```python
from build123d import *

# Parameters (mm, degrees)
F0_W     = 103.353604
F0_H     = 45.458422
F1_DEPTH = 25.4
F2_R     = 12.877415
F3_R     = 21.377303
F4_DEPTH = 27.686


with BuildPart() as f1:
    # F0 (on Top) → F1 (new body)
    with BuildSketch(Plane.XY):
        Rectangle(F0_W, F0_H)
    extrude(amount=F1_DEPTH)

    # F2
    f2_edges = [f1.edges().sort_by_distance(p)[0] for p in [
        (51.676802, 22.729211, 12.7),
        (51.676802, -22.729211, 12.7),
    ]]
    fillet(f2_edges, radius=F2_R)

    # F3 (on Top) → F4 (join)
    with BuildSketch(Plane.XY):
        with Locations((-21.615615, 0)):
            Circle(F3_R)
    extrude(amount=-F4_DEPTH)


solid = f1.part
```
The listing builds one solid part. Answer for the finished solid, in the listing's coordinates (mm). A direction names the side the tool comes from. Round coordinates to 2 decimals unless told otherwise and drop trailing zeros. Loops run counter-clockwise (first coordinate to the right, second up) from the corner with the lowest first, then second, coordinate; pieces in that order, holes last.
Q1. Section C-C, the plane x = -28.5 is taken. Determine the outline of the cut face in (y, z), then the cut area to 3 significant figures.
Q2. Section B-B, the plane z = -9 is taken. Determine the outline of the cut face in (x, y), then the cut area to 3 significant figures.
Q3. Find the intervals of material crossed by line 1 (Z direction, x = 26.5, y = -10); line 2 (X direction, y = -0.5, z = -16); line 3 (X direction, y = 16.5, z = -7), in increasing order.
Q4. Given pin 1 Ø2 at (y, z) = (11.5, 8) entering from +X; pin 2 Ø13.5 at (x, y) = (18, 4.5) entering from -Z; pin 3 Ø12 at (x, z) = (-32.5, -16.5) entering from +Y; pin 4 Ø12 at (x, z) = (18.5, -7.5) entering from +Y, each flat-ended and moving along its own axis, determine where each tip first touches the part or whether it passes through.
Q5. Section D-D, the plane x = 16 is taken. Determine the outline of the cut face in (y, z).
Q6. Section A-A, the plane y = 0 is taken. Determine the outline of the cut face in (x, z), then the cut area to 3 significant figures.
Q7. Which of the six approach directions +Z, -Z, +X, -X, +Y, -Y give full straight-line access (tool end or side, diameter ignored) to faces 1 (the face through (-11.751, -18.965, -13.649)), 2 (the face through (48, 18.86, 12.88))?
Completed:
1. outline: (-22.73, 0) - (-20.24, 0) - (-20.24, -27.69) - (20.24, -27.69) - (20.24, 0) - (22.73, 0) - (22.73, 25.4) - (-22.73, 25.4) - close
1. area: 2,280 mm2
2. outline: circle Ø42.75 at (-21.62, 0)
2. area: 1,440 mm2
3. line 1: z = 0 to 25.4
3. line 2: x = -42.99 to -0.24
3. line 3: x = -35.21 to -8.02
4. pin 1: stops at x = 51.66
4. pin 2: stops at z = 0
4. pin 3: stops at y = 20.81
4. pin 4: passes through
5. outline: (-22.73, 0) - (22.73, 0) - (22.73, 25.4) - (-22.73, 25.4) - close
6. outline: (-51.68, 0) - (-42.99, 0) - (-42.99, -27.69) - (-0.24, -27.69) - (-0.24, 0) - (51.68, 0) - (51.68, 25.4) - (-51.68, 25.4) - close
6. area: 3,810 mm2
7. face 1: -Z
7. face 2: +Z, -Z, +X, +Y
